The listing builds one solid part. Answer for the finished solid, in the listing's coordinates (mm). Face numbers are marked on the shaded views. A direction names the side the tool comes from. Round coordinates to 2 decimals unless told otherwise and drop trailing zeros. Order: outer loops, then holes, each group sorted by start corner. A loop starts at its lowest first (then second) coordinate and runs counter-clockwise, first axis right, second up. Notation, with made-up numbers: (38, 34.25) - (43, 34.25) arc R32 ccw to (43, 67.25) - close; hole circle Ø2 at (17, 16). An arc over 180 degrees is marked (long way). One line per item, written item: value. Start each with the question number.
1. Straight lines are drawn through the part: line 1 (Z direction, x = 0.85, y = 0); line 2 (X direction, y = 4, z = 0.5); line 3 (Z direction, x = 1.5, y = -0.75). For each, find the intervals that lie inside material, in ascending order.
2. A tool of negligible diameter and unlimited length cuts with its end or side. For the marked faces 4 and 5, from which of +Z, -Z, +X, -X, +Y, -Y can it reach the whole face along a straight path? Write none if from no direction.
3. For a pull along Z with two mould halves and no side action, classify the marked faces 1, 2 and 3 as released by +Z, released by -Z, zero draft, split by the parting line, or undercut.
4. Section A-A, the plane y = 0 is taken. Give the vertices of the cut face in (x, z) (3 decimals), then the cut area to 3 significant figures.
5. Flat-ended cylindrical pins translate along their axes: P1, Ø1, axis at x = 0.5, z = -2.5, coming from the +Y side; P2, Ø1.5, axis at x = 0.5, y = -1, coming from the -Z side; P3, Ø1.5, axis at x = 1.5, z = -0.5, coming from the -Y side; P4, Ø2.5, axis at y = 0, z = 0, coming from the -X side. Find the tip coordinate at first contact, or state that the pin passes through.
6. Section C-C, the plane x = 1.65 is taken. Give the vertices of the cut face in (y, z).
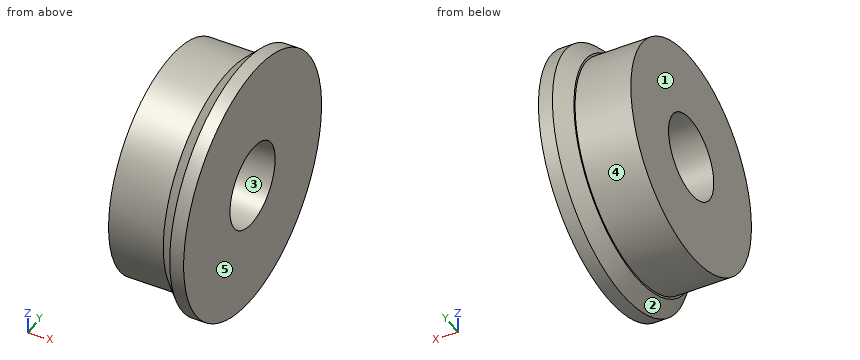
Autodesk Inventor part; units mm, degrees
ref_plane "YZ Plane" through (0, 0, 0) normal (1, 0, 0) x (0, 1, 0)
ref_plane "XZ Plane" through (0, 0, 0) normal (0, 1, 0) x (-1, 0, 0)
ref_plane "XY Plane" through (0, 0, 0) normal (0, 0, 1) x (1, 0, 0)
sketch "Skizze1" plane through (0, 0, 0) normal (1, 0, 0) x (0, 1, 0)
  circle A0 centre (0, 0) radius 4
  circle A1 centre (0, 0) radius 1.5
  dimension "d0" = 8
  dimension "d1" = 3
extrude "Extrusion1" add sketch "Skizze1" along normal blind 2
sketch "Skizze2" plane through (2, 0, 0) normal (1, 0, 0) x (0, 0, -1)
  circle A0 centre (0, 0) radius 4
  circle A1 centre (0, 0) radius 1.5
  circle A2 centre (0, 0) radius 4.575
  dimension "d4" = 9.15
extrude "Extrusion2" add sketch "Skizze2" along normal blind 1 contours A0 | A2
chamfer "Fase1" distance 0.5 angle 45 1 edges at (2, 0, 4.575)
properties part number "00_Bearing_8mm"
Answer list:
1. line 1: z = -4 to -1.5, 1.5 to 4
1. line 2: x = 2 to 3
1. line 3: z = -3.93 to -1.3, 1.3 to 3.93
2. face 4: -X
2. face 5: +Z, -Z, +X, +Y, -Y
3. face 1: zero draft
3. face 2: split by the parting line
3. face 3: undercut
4. outline: (0, -4) - (2, -4) - (2, -4.075) - (2.5, -4.575) - (3, -4.575) - (3, -1.5) - (0, -1.5) - close; (0, 1.5) - (3, 1.5) - (3, 4.575) - (2.5, 4.575) - (2, 4.075) - (2, 4) - (0, 4) - close
4. area: 15.9 mm²
5. P1: stops at y = 3.46
5. P2: stops at z = -3.99
5. P3: stops at y = -4.3
5. P4: passes through
6. outline: circle Ø8 at (0, 0); hole circle Ø3 at (0, 0)
